Source: CAD feature listing. Evaluate the final solid. Frame: model axes, mm. Face numbers are marked on the shaded views. Give positions to 0.01 mm unless a question says otherwise; leave off trailing zeros. Order: outer loops, then holes, each group sorted by start corner. A loop starts at its lowest first (then second) coordinate and runs counter-clockwise, first axis right, second up. Notation, with made-up numbers: M 27,36.25 L 37,36.25 A26 ccw 37,51.25 Z; hole C -5,52 d10. An arc over 180 degrees is marked long. Answer as a JSON object with one key per item and string values. Group by question number.
1. Section query A-A (y = 51). Output: boundary loops of the cut face in (x, z), plus the area to 4 significant figures.
2. Material intervals for L1, parallel to Y at x = 83, z = 7.75; L2, parallel to X at y = 86.5, z = 3.5, sorted ascending. Write a range as [from, to].
3. Pin query (flat end, axial travel): P1, Ø5, axis at y = 34, z = 11, coming from the -X side; P2, Ø2.5, axis at x = 86, y = 52.5, coming from the -Z side. Return the tip coordinate at first contact, or that it passes through.
4. Pull-direction query (Y, two-part tool) for the marked faces 1, 2, 3 and 4; classes: +Y half, -Y half, draft (parallel to the pull), parting line (faces both ways), or undercut.
5. Section query B-B (z = 7.75). Count the separate pieces of the cut face and the enclosed holes in it, plus the area to 3 significant figures.
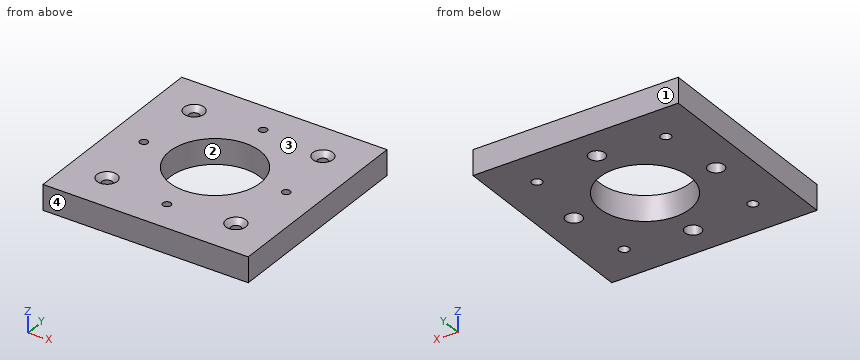
from build123d import *

# Parameters (mm, degrees)
F3_W           = 102
F3_H           = 102
F4_DEPTH       = 12.5
F5_D           = 45
F1_D           = 5
F1_CSINK_D     = 10
F1_CSINK_ANGLE = 90
F2_D           = 5
F2_CSINK_D     = 10
F2_CSINK_ANGLE = 90
F8_D           = 4
F8_CBORE_D     = 8
F8_CBORE_DEPTH = 5


with BuildPart() as f4:
    # F3 (on Top) → F4 (new body)
    with BuildSketch(Plane.XY):
        with Locations((51, 51)):
            Rectangle(F3_W, F3_H)
    extrude(amount=F4_DEPTH)

    # F5 (through all)
    with Locations(Plane.XY.offset(12.5)):
        with Locations((51, 51)):
            Hole(F5_D / 2)

    # F1 (through all)
    with Locations(Plane.XY.offset(12.5)):
        with Locations((19, 19)):
            CounterSinkHole(F1_D / 2, F1_CSINK_D / 2, counter_sink_angle=F1_CSINK_ANGLE)

    # F2 (through all)
    with Locations(Plane.XY.offset(12.5)):
        with Locations((83, 83), (19, 83), (83, 19)):
            CounterSinkHole(F2_D / 2, F2_CSINK_D / 2, counter_sink_angle=F2_CSINK_ANGLE)

    # F8 (through all)
    with Locations(Plane(origin=(0, 0, 0), x_dir=(1, 0, 0), z_dir=(0, 0, -1))):
        with Locations((15.644661, -51), (51, -15.644661), (86.355339, -51), (51, -86.355339)):
            CounterBoreHole(F8_D / 2, F8_CBORE_D / 2, F8_CBORE_DEPTH)


solid = f4.part
Answer sheet:
{
 "1": {"outline": "M 0,0 L 11.64,0 L 11.64,5 L 13.64,5 L 13.64,12.5 L 0,12.5 Z; M 17.64,5 L 19.64,5 L 19.64,0 L 28.5,0 L 28.5,12.5 L 17.64,12.5 Z; M 73.5,0 L 82.36,0 L 82.36,5 L 84.36,5 L 84.36,12.5 L 73.5,12.5 Z; M 88.36,5 L 90.36,5 L 90.36,0 L 102,0 L 102,12.5 L 88.36,12.5 Z", "area": "572.5 mm^2"},
 "2": {"L1": "[0, 16.5], [21.5, 80.5], [85.5, 102]", "L2": "[0, 47], [55, 102]"},
 "3": {"P1": "x = 0", "P2": "z = 5"},
 "4": {"face 1": "+Y half", "face 2": "undercut", "face 3": "draft", "face 4": "-Y half"},
 "5": {"separate pieces": "1", "enclosed holes": "9", "area": "8,680 mm^2"}
}
